CAD build for the part. Positions are in the model's coordinates, mm. A direction names the side the tool comes from. Coordinates: 2 decimals unless noted, no trailing zeros. Loops run counter-clockwise (first coordinate to the right, second up) from the corner with the lowest first, then second, coordinate; pieces in that order, holes last. Notation, with made-up numbers: (-10.75, -3) -> (22.25, -3) arc R9 ccw to (22.25, 1) -> close; hole circle Ø6 at (88.25, 23). An arc over 180 degrees is marked (long way). Answer as a JSON object with one key per item and string values. Group by question number.
from build123d import *

# Parameters (mm, degrees)
ESQUISSE1_W              = 280.2
ESQUISSE1_H              = 276.282873123
BOSS_EXTRU_1_DEPTH       = 5
ENL_V_MAT_EXTRU_1_DEPTH  = 6
ENL_V_MAT_EXTRU_3_DEPTH  = 6
ESQUISSE5_R              = 2
ENL_V_MAT_EXTRU_4_DEPTH  = 6
ENL_V_MAT_EXTRU_5_DEPTH  = 6
ESQUISSE7_R              = 7.071067812
ENL_V_MAT_EXTRU_6_DEPTH  = 6
ESQUISSE8_R              = 1.5
ENL_V_MAT_EXTRU_8_DEPTH  = 6
ESQUISSE9_R              = 32.5
ENL_V_MAT_EXTRU_10_DEPTH = 3
ESQUISSE10_R             = 1.5
ENL_V_MAT_EXTRU_11_DEPTH = 6


with BuildPart() as part:
    # Esquisse1 → Boss.-Extru.1 (new body)
    with BuildSketch(Plane(origin=(0, 0, 0), x_dir=(1, 0, 0), z_dir=(0, 1, 0))):
        with Locations((0, -106.941436562)):
            Rectangle(ESQUISSE1_W, ESQUISSE1_H)
    extrude(amount=BOSS_EXTRU_1_DEPTH)

    # Esquisse2 → Enlèv. mat.-Extru.1 (cut, through all)
    with BuildSketch(Plane(origin=(0, 5, 0), x_dir=(1, 0, 0), z_dir=(0, 1, 0))):
        with BuildLine():
            Line((-86.286307054, -217.873386842), (-88.029045643, -220.315284098))
            ThreePointArc((-88.029045643, -220.315284098), (-128.330678708, -98.90890093), (-25, -23.5))
            ThreePointArc((-25, -23.5), (78.330678708, -98.90890093), (38.029045643, -220.315284098))
            Line((38.029045643, -220.315284098), (36.286307054, -217.873386842))
            ThreePointArc((36.286307054, -217.873386842), (30.714652713, -234.657679446), (45, -245.082873123))
            Line((45, -245.082873123), (-95, -245.082873123))
            ThreePointArc((-95, -245.082873123), (-80.714652713, -234.657679446), (-86.286307054, -217.873386842))
        make_face()
    extrude(amount=-ENL_V_MAT_EXTRU_1_DEPTH, mode=Mode.SUBTRACT)

    # Esquisse4 → Enlèv. mat.-Extru.3 (cut, through all)
    with BuildSketch(Plane(origin=(0, 5, 0), x_dir=(1, 0, 0), z_dir=(0, 1, 0))):
        with BuildLine():
            Line((140.1, -245.082873123), (101.1, -245.082873123))
            ThreePointArc((101.1, -245.082873123), (128.677164466, -233.660037589), (140.1, -206.082873123))
            Line((140.1, -206.082873123), (140.1, -245.082873123))
        make_face()
        with BuildLine():
            Line((-101.1, -245.082873123), (-140.1, -245.082873123))
            Line((-140.1, -245.082873123), (-140.1, -206.082873123))
            ThreePointArc((-140.1, -206.082873123), (-128.677164466, -233.660037589), (-101.1, -245.082873123))
        make_face()
    extrude(amount=-ENL_V_MAT_EXTRU_3_DEPTH, mode=Mode.SUBTRACT)

    # Esquisse5 → Enlèv. mat.-Extru.4 (cut, through all)
    with BuildSketch(Plane(origin=(0, 5, 0), x_dir=(1, 0, 0), z_dir=(0, 1, 0))):
        with Locations((-91, -232)):
            Circle(ESQUISSE5_R)
        with Locations((41, -232)):
            Circle(ESQUISSE5_R)
    extrude(amount=-ENL_V_MAT_EXTRU_4_DEPTH, mode=Mode.SUBTRACT)

    # Esquisse6 → Enlèv. mat.-Extru.5 (cut, through all)
    with BuildSketch(Plane(origin=(0, 5, 0), x_dir=(1, 0, 0), z_dir=(0, 1, 0))):
        with BuildLine():
            Line((140.1, 31.2), (0, 31.2))
            Line((0, 31.2), (-140.1, 31.2))
            Line((-140.1, 31.2), (-140.1, -41.25))
            ThreePointArc((-140.1, -41.25), (-138.635533906, -37.714466094), (-135.1, -36.25))
            Line((-135.1, -36.25), (-128.5, -36.25))
            ThreePointArc((-128.5, -36.25), (-124.964466094, -34.785533906), (-123.5, -31.25))
            Line((-123.5, -31.25), (-123.5, -21.2))
            Line((-123.5, -21.2), (-113.5, -21.2))
            Line((-113.5, -21.2), (-113.5, -28.25))
            ThreePointArc((-113.5, -28.25), (-112.035533906, -31.785533906), (-108.5, -33.25))
            Line((-108.5, -33.25), (-104.5, -33.25))
            ThreePointArc((-104.5, -33.25), (-100.964466094, -31.785533906), (-99.5, -28.25))
            Line((-99.5, -28.25), (-99.5, -24))
            ThreePointArc((-99.5, -24), (-98.035533906, -20.464466094), (-94.5, -19))
            Line((-94.5, -19), (-58.5, -19))
            ThreePointArc((-58.5, -19), (-54.964466094, -17.535533906), (-53.5, -14))
            Line((-53.5, -14), (-53.5, 21.2))
            Line((-53.5, 21.2), (53.5, 21.2))
            Line((53.5, 21.2), (53.5, -14))
            ThreePointArc((53.5, -14), (54.964466094, -17.535533906), (58.5, -19))
            Line((58.5, -19), (94.5, -19))
            ThreePointArc((94.5, -19), (98.035533906, -20.464466094), (99.5, -24))
            Line((99.5, -24), (99.5, -28.25))
            ThreePointArc((99.5, -28.25), (100.964466094, -31.785533906), (104.5, -33.25))
            Line((104.5, -33.25), (108.5, -33.25))
            ThreePointArc((108.5, -33.25), (112.035533906, -31.785533906), (113.5, -28.25))
            Line((113.5, -28.25), (113.5, -21.2))
            Line((113.5, -21.2), (123.5, -21.2))
            Line((123.5, -21.2), (123.5, -31.25))
            ThreePointArc((123.5, -31.25), (124.964466094, -34.785533906), (128.5, -36.25))
            Line((128.5, -36.25), (135.1, -36.25))
            ThreePointArc((135.1, -36.25), (138.635533906, -37.714466094), (140.1, -41.25))
            Line((140.1, -41.25), (140.1, 31.2))
        make_face()
    extrude(amount=-ENL_V_MAT_EXTRU_5_DEPTH, mode=Mode.SUBTRACT)

    # Esquisse7 → Enlèv. mat.-Extru.6 (cut, through all)
    with BuildSketch(Plane(origin=(0, 5, 0), x_dir=(1, 0, 0), z_dir=(0, 1, 0))):
        with Locations((-118.5, -215.8)):
            Circle(ESQUISSE7_R)
    extrude(amount=-ENL_V_MAT_EXTRU_6_DEPTH, mode=Mode.SUBTRACT)

    # Esquisse8 → Enlèv. mat.-Extru.8 (cut, through all)
    with BuildSketch(Plane.XZ):
        with Locations((47.5, -16.2)):
            Circle(ESQUISSE8_R)
        with Locations((-47.5, -16.2)):
            Circle(ESQUISSE8_R)
    extrude(amount=-ENL_V_MAT_EXTRU_8_DEPTH, mode=Mode.SUBTRACT)

    # Esquisse9 → Enlèv. mat.-Extru.10 (cut)
    with BuildSketch(Plane(origin=(0, 5, 0), x_dir=(1, 0, 0), z_dir=(0, 1, 0))):
        with Locations((101.1, -206.082873123)):
            Circle(ESQUISSE9_R)
    extrude(amount=-ENL_V_MAT_EXTRU_10_DEPTH, mode=Mode.SUBTRACT)

    # Esquisse10 → Enlèv. mat.-Extru.11 (cut, through all)
    with BuildSketch(Plane(origin=(0, 5, 0), x_dir=(1, 0, 0), z_dir=(0, 1, 0))):
        with Locations((118.5, -57.265046493)):
            Circle(ESQUISSE10_R)
        with Locations((-118.5, -57.265046493)):
            Circle(ESQUISSE10_R)
    extrude(amount=-ENL_V_MAT_EXTRU_11_DEPTH, mode=Mode.SUBTRACT)


solid = part.part
Item 1: Pull direction Z, two halves, no side cores. Call faces 1 (the flat face through (101, 2, 206)), 2 (the flat face through (82, 5, 92)), 3 (the cylindrical face through (-128.979, 2.535, 233.355)): +Z half, -Z half, draft (parallel to the pull), parting line (faces both ways), or undercut.
Item 2: Band-saw the part on C-C, the plane x = 6.5. List the corners of the cut face in (y, z), and give its area (3 significant figures).
Item 3: Band-saw the part on D-D, the plane z = 89. List the corners of the cut face in (x, y).
Item 4: Flat gauge pins, fed straight in: P1, Ø12.5, axis at x = -118.5, z = 215.8, coming from the +Y side; P2, Ø1.5, axis at x = -120, y = 2, coming from the -Z side; P3, Ø2.5, axis at x = -74, y = 2.5, coming from the -Z side; P4, Ø1.5, axis at x = -132, y = 3.5, coming from the -Z side. Where does each tip first touch, or does it go through?
Item 5: Band-saw the part on B-B, the plane z = 0. List the corners of the cut face in (x, y).
Item 6: 3-axis set-ups, long thin cutter, end or side, ignore diameter. For faces 4 (the flat face through (60, 0, 51)), 5 (the cylindrical face through (30.636, 2.535, 234.405)), 6 (the cylindrical face through (131.12, 3.52, 218.53)): which of +Z, -Z, +X, -X, +Y, -Y reach the whole face in a straight line?
Item 7: Band-saw the part on A-A, the plane z = 132. List the corners of the cut face in (x, y), and give its area (3 significant figures).
Item 8: Drill centre lines: L1, parallel to X at y = 3.95, z = 232; L2, parallel to X at y = 1.75, z = 215.8; L3, parallel to Z at x = -92, y = 2.45. Where is each one in solid material? Low to high.
Reply:
{
 "1": {"face 1": "undercut", "face 2": "draft", "face 3": "+Z half"},
 "2": {"outline": "(0, -21.2) -> (5, -21.2) -> (5, 28.17) -> (0, 28.17) -> close", "area": "247 mm²"},
 "3": {"outline": "(-140.1, 0) -> (-124.62, 0) -> (-124.62, 5) -> (-140.1, 5) -> close; (74.62, 0) -> (140.1, 0) -> (140.1, 5) -> (74.62, 5) -> close"},
 "4": {"P1": "through", "P2": "z = 21.2", "P3": "z = 19", "P4": "z = 36.25"},
 "5": {"outline": "(-53.5, 0) -> (53.5, 0) -> (53.5, 5) -> (-53.5, 5) -> close"},
 "6": {"face 4": "+Z, -Z, +X, -X, -Y", "face 5": "+Y, -Y", "face 6": "+Y"},
 "7": {"outline": "(-140.1, 0) -> (-133.5, 0) -> (-133.5, 5) -> (-140.1, 5) -> close; (83.5, 0) -> (140.1, 0) -> (140.1, 5) -> (83.5, 5) -> close", "area": "316 mm²"},
 "8": {"L1": "-130.24 to -93, -89 to -80.12, 30.12 to 39, 43 to 81.49, 120.71 to 130.24", "L2": "-138.87 to -125.57, -111.43 to -93.92, 43.92 to 138.87", "L3": "19 to 46.66, 217.34 to 230.27, 233.73 to 244.78"}
}
